Could you check a few things on this drawing? It's one solid part, dimensions in mm from its lowest x, y, z. A direction names the side the tool comes from. Give positions to 0.01 mm unless a question says otherwise; leave off trailing zeros. Order: outer loops, then holes, each group sorted by start corner. A loop starts at its lowest first (then second) coordinate and runs counter-clockwise, first axis right, second up.
(1) Imagine slicing it at B-B, the plane z = 12.5. Write out the boundary of the cut face in (x, y) (3 decimals).
(2) Imagine slicing it at D-D, the plane z = 4.5. Write out the boundary of the cut face in (x, y) (1 decimal).
(3) Imagine slicing it at A-A, the plane x = 12.54. Write out the boundary of the cut face in (y, z) (1 decimal).
(4) Will these pins go through, and if not, where does the flat tip stop? pin 1 (7.5 mm diameter, centred on x = 18.5, z = 22.5, fed in from -Y) (3 decimals); pin 2 (6.5 mm diameter, centred on x = 3.5, z = 14.5, fed in from +Y); pin 3 (1.6 mm diameter, centred on y = 3, z = 28.5, fed in from +X) (3 decimals).
(5) If I drill on probe 1 along Z at (x, y) = (12.54, 3.85); probe 2 along X at (y, z) = (0.6, 4) (3 decimals); probe 3 along X at (y, z) = (2.7, 29.5) (3 decimals), over which ranges is the centre line in solid material (lowest first)?
(6) Imagine slicing it at C-C, the plane y = 4. Write out the boundary of the cut face in (x, z) (1 decimal), then the cut area to 3 significant figures.
(7) On a 3-axis mill with a long thin cutter (end or side, diameter ignored), from which of +Z, -Z, +X, -X, +Y, -Y can I reach the whole of each face in a straight line? I mean the marked faces 1, 2 and 3. Say none if no direction works.
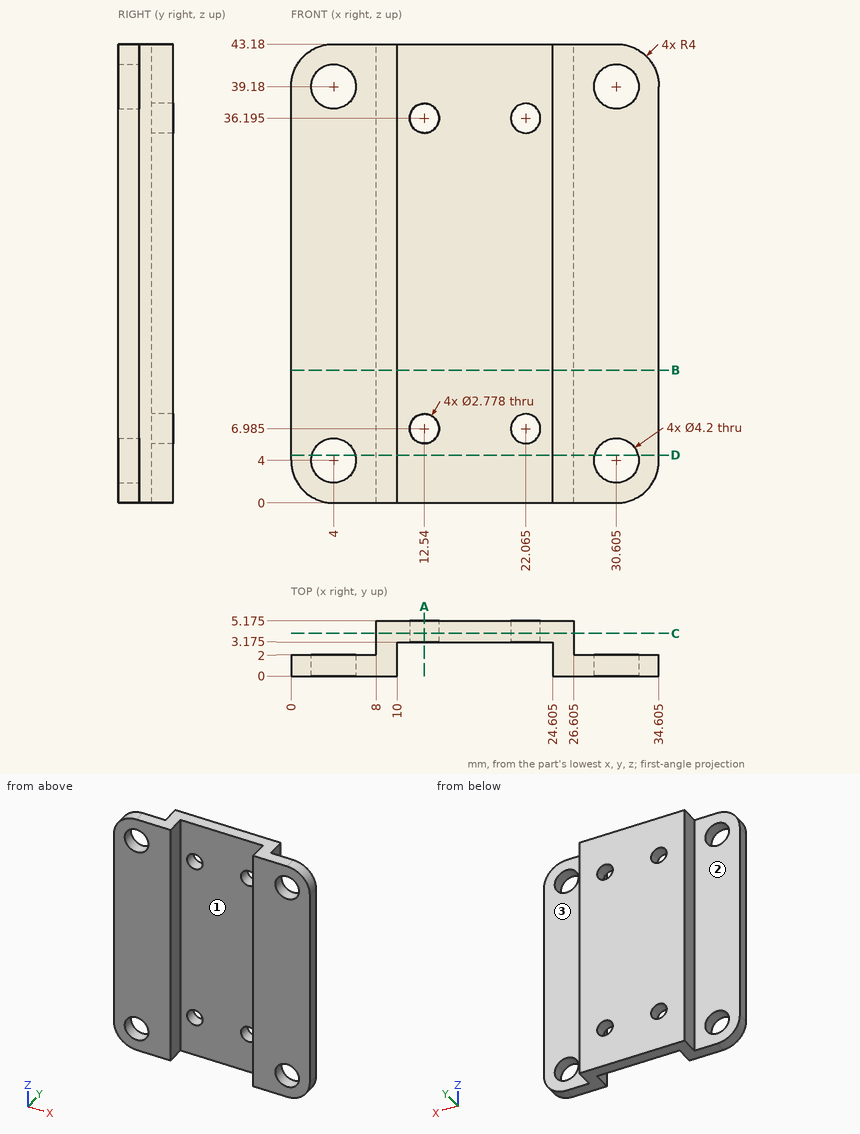
Answer block:
1. outline: (0, 0) - (10, 0) - (10, 3.175) - (24.605, 3.175) - (24.605, 0) - (34.605, 0) - (34.605, 2) - (26.605, 2) - (26.605, 5.175) - (8, 5.175) - (8, 2) - (0, 2) - close
2. outline: (0, 0) - (2, 0) - (2, 2) - (0, 2) - close; (6, 0) - (10, 0) - (10, 3.2) - (24.6, 3.2) - (24.6, 0) - (28.6, 0) - (28.6, 2) - (26.6, 2) - (26.6, 5.2) - (8, 5.2) - (8, 2) - (6, 2) - close; (32.6, 0) - (34.6, 0) - (34.6, 2) - (32.6, 2) - close
3. outline: (3.2, 0) - (5.2, 0) - (5.2, 5.6) - (3.2, 5.6) - close; (3.2, 8.4) - (5.2, 8.4) - (5.2, 34.8) - (3.2, 34.8) - close; (3.2, 37.6) - (5.2, 37.6) - (5.2, 43.2) - (3.2, 43.2) - close
4. pin 1: stops at y = 3.175
4. pin 2: stops at y = 2
4. pin 3: stops at x = 26.605
5. probe 1: z = 0 to 5.6, 8.37 to 34.81, 37.58 to 43.18
5. probe 2: x = 0 to 1.9, 6.1 to 10, 24.605 to 28.505, 32.705 to 34.605
5. probe 3: x = 8 to 10, 24.605 to 26.605
6. outline: (8, 0) - (26.6, 0) - (26.6, 43.2) - (8, 43.2) - close; hole circle Ø2.8 at (12.5, 7); hole circle Ø2.8 at (12.5, 36.2); hole circle Ø2.8 at (22.1, 7); hole circle Ø2.8 at (22.1, 36.2)
6. area: 779 mm2
7. face 1: +Z, -Z, -Y
7. face 2: +Z, -Z, -X, +Y
7. face 3: +Z, -Z, +X, +Y
